from build123d import *

# Parameters (mm, degrees)
IZIM1_R                          = 7.5
Y_KSEKLIK_EKSTR_ZYON1_DEPTH      = 15
Y_KSEKLIK_EKSTR_ZYON2_DEPTH      = 5
Y_KSEKLIK_EKSTR_ZYON2_DEPTH_BACK = 5
IZIM2_W                          = 15
IZIM2_H                          = 38.236646402
RADYUS1_R                        = 10
RADYUS2_R                        = 2
IZIM3_R                          = 3.5
KES_EKSTR_ZYON1_DEPTH            = 10
IZIM4_W                          = 40
IZIM4_H                          = 20
Y_KSEKLIK_EKSTR_ZYON3_DEPTH      = 5


with BuildPart() as part:
    # Çizim1 → Yükseklik-Ekstrüzyon1 (new body)
    with BuildSketch(Plane.XY):
        with Locations((0, 31.714285714)):
            Circle(IZIM1_R)
    extrude(amount=Y_KSEKLIK_EKSTR_ZYON1_DEPTH)

    # Çizim2 → Yükseklik-Ekstrüzyon2 (add, two sides: drawn at the far end of the back side and taken through both)
    with BuildSketch(Plane.XY.offset(15).offset(-Y_KSEKLIK_EKSTR_ZYON2_DEPTH_BACK)):
        with Locations((0, 12.595962513)):
            Rectangle(IZIM2_W, IZIM2_H)
    extrude(amount=Y_KSEKLIK_EKSTR_ZYON2_DEPTH + Y_KSEKLIK_EKSTR_ZYON2_DEPTH_BACK)

    # Radyus1
    # the kernel refuses this fillet: 10 mm, written as the material it adds along each edge
    with BuildSketch(Plane(origin=(29.150635095, 31.714285714, 15), x_dir=(0, 1, 0), z_dir=(-1, 0, 0))) as radyus1_piece_1_section:
        with BuildLine():
            CenterArc((8.660254038, -10), RADYUS1_R, 90, 60)
            Line((0, -5), (0, 0))
            Line((0, 0), (8.660254038, 0))
        make_face()
    radyus1_piece_1 = extrude(amount=58.301270189, mode=Mode.PRIVATE)
    radyus1_piece_1 = radyus1_piece_1 & Plane(origin=(0, 31.714285714, 15), x_dir=(1, 0, 0), z_dir=(0, 0, -1)) * Cylinder(7.5, 152, mode=Mode.PRIVATE)
    add(radyus1_piece_1)

    # Radyus2
    # the kernel refuses this fillet: 2 mm, written as the material it takes off along each edge
    with BuildSketch(Plane(origin=(-7.5, -11.522360688, 10), x_dir=(0, 0, 1), z_dir=(0, 1, 0))) as radyus2_piece_1_section:
        with BuildLine():
            CenterArc((RADYUS2_R, RADYUS2_R), RADYUS2_R, 180, 90)
            Line((0, RADYUS2_R), (0, 0))
            Line((0, 0), (RADYUS2_R, 0))
        make_face()
    radyus2_piece_1 = extrude(amount=51.736646403, mode=Mode.PRIVATE)
    radyus2_piece_1 = radyus2_piece_1 - Plane(origin=(0, 31.714285714, 10), x_dir=(1, 0, 0), z_dir=(0, 0, -1)) * Cylinder(7.5, 112, mode=Mode.PRIVATE)
    add(radyus2_piece_1, mode=Mode.SUBTRACT)
    with BuildSketch(Plane(origin=(-7.5, -11.522360688, 20), x_dir=(0, 0, -1), z_dir=(0, 1, 0)), Plane(origin=(7.5, 40.214285714, 20), x_dir=(0, 0, -1), z_dir=(0, -1, 0))) as radyus2_piece_2:
        with BuildLine():
            CenterArc((RADYUS2_R, -RADYUS2_R), RADYUS2_R, 90, 90)
            Line((0, -RADYUS2_R), (0, 0))
            Line((0, 0), (RADYUS2_R, 0))
        make_face()
    extrude(amount=51.736646403, mode=Mode.SUBTRACT)
    with BuildSketch(Plane(origin=(7.5, 40.214285714, 10), x_dir=(-1, 0, 0), z_dir=(0, -1, 0))) as radyus2_piece_3_section:
        with BuildLine():
            CenterArc((RADYUS2_R, -RADYUS2_R), RADYUS2_R, 90, 90)
            Line((0, -RADYUS2_R), (0, 0))
            Line((0, 0), (RADYUS2_R, 0))
        make_face()
    radyus2_piece_3 = extrude(amount=51.736646403, mode=Mode.PRIVATE)
    radyus2_piece_3 = radyus2_piece_3 - Plane(origin=(0, 31.714285714, 10), x_dir=(1, 0, 0), z_dir=(0, 0, -1)) * Cylinder(7.5, 112, mode=Mode.PRIVATE)
    add(radyus2_piece_3, mode=Mode.SUBTRACT)

    # Çizim3 → Kes-Ekstrüzyon1 (cut)
    with BuildSketch(Plane(origin=(0, 0, 0), x_dir=(-1, 0, 0), z_dir=(0, 0, -1))):
        with Locations((0, 31.714285714)):
            Circle(IZIM3_R)
    extrude(amount=-KES_EKSTR_ZYON1_DEPTH, mode=Mode.SUBTRACT)

    # Çizim4 → Yükseklik-Ekstrüzyon3 (add)
    with BuildSketch(Plane(origin=(0, -6.522360688, 0), x_dir=(-1, 0, 0), z_dir=(0, -1, 0))):
        with Locations((0.752019729, -14.638510347)):
            Rectangle(IZIM4_W, IZIM4_H)
    extrude(amount=Y_KSEKLIK_EKSTR_ZYON3_DEPTH)


solid = part.part
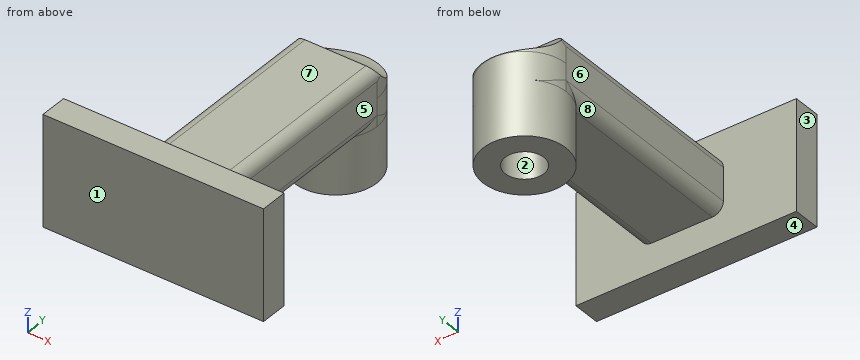
The model under review builds one solid part; all positions refer to its coordinate system, in mm. Face numbers are marked on the shaded views. A direction names the side the tool comes from. Round coordinates to 2 decimals unless told otherwise and drop trailing zeros. Loops run counter-clockwise (first coordinate to the right, second up) from the corner with the lowest first, then second, coordinate; pieces in that order, holes last. Notation, with made-up numbers: (-1.5, -37.5) -> (36.5, -37.5) arc R30 ccw to (36.5, 0.5) -> close; hole circle Ø2 at (-8.5, 7). An arc over 180 degrees is marked (long way). One line per question, with ' | ' between items. Start each with the question number.
Item 1: Draft analysis for pull direction Y (two halves, no side actions). For the marked faces 1, 2 and 3, state which applies: +Y half, -Y half, draft (parallel to the pull), parting line (faces both ways), or undercut.
Item 2: Wall thickness on line 1 along Y through (x, z) = (0, 4.75); line 2 along Y through (x, z) = (0, 2.75); line 3 along X through (y, z) = (31.5, 3.5): over which ranges is each line inside the solid? List them lowest first. Write a range as [from, to].
Item 3: Add section D-D, the plane z = 16.75. Write out the cut boundary in (x, y).
Item 4: Add section B-B, the plane y = 19. Write out the cut boundary in (x, z).
Item 5: Add section C-C, the plane x = 0. Write out the cut boundary in (y, z).
Item 6: For pin 1 (1.8 mm diameter, centred on y = 18.5, z = 15, fed in from -X); pin 2 (4 mm diameter, centred on x = -5.5, y = -9.5, fed in from -Z); pin 3 (8 mm diameter, centred on x = 0, y = 31.71, fed in from +Z), all flat-tipped, find the tip position at first contact; note any pin that passes through.
Item 7: Add section A-A, the plane z = 5.5. Write out the cut boundary in (x, y).
Item 8: Machinability: for the marked faces 4, 5, 6, 7 and 8, which of the approach directions +Z, -Z, +X, -X, +Y, -Y give a long, thin tool a straight path to every point of the face, cutting with its end or side? Answer none if there is none.
Return value:
1) face 1: -Y half | face 2: undercut | face 3: draft
2) line 1: y = [-11.52, -6.52], [24.21, 28.21], [35.21, 39.21] | line 2: y = [24.21, 28.21], [35.21, 39.21] | line 3: x = [-7.5, -3.49], [3.49, 7.5]
3) outline: (-20.75, -11.52) -> (19.25, -11.52) -> (19.25, -6.52) -> (7.5, -6.52) -> (7.5, 31.71) arc R7.5 ccw to (6.87, 34.72) -> (-6.87, 34.72) arc R7.5 ccw to (-7.5, 31.71) -> (-7.5, -6.52) -> (-20.75, -6.52) -> close
4) outline: (-7.5, 12) arc R2 ccw to (-5.5, 10) -> (5.5, 10) arc R2 ccw to (7.5, 12) -> (7.5, 18) arc R2 ccw to (5.5, 20) -> (-5.5, 20) arc R2 ccw to (-7.5, 18) -> close
5) outline: (-11.52, 4.64) -> (-6.52, 4.64) -> (-6.52, 10) -> (24.21, 10) -> (24.21, 0) -> (28.21, 0) -> (28.21, 10) -> (35.21, 10) -> (35.21, 0) -> (39.21, 0) -> (39.21, 15.07) arc R10 cw to (31.71, 20) -> (-6.52, 20) -> (-6.52, 24.64) -> (-11.52, 24.64) -> close
6) pin 1: stops at x = -7.5 | pin 2: stops at z = 4.64 | pin 3: stops at z = 20
7) outline: (-20.75, -11.52) -> (19.25, -11.52) -> (19.25, -6.52) -> (-20.75, -6.52) -> close; circle Ø15 at (0, 31.71); hole circle Ø7 at (0, 31.71)
8) face 4: -Z, +X, -X, -Y | face 5: +Z, -Z, +X, +Y | face 6: +Z, -Z, -X, +Y | face 7: +Z, +X, -X, +Y | face 8: -Z, -X
